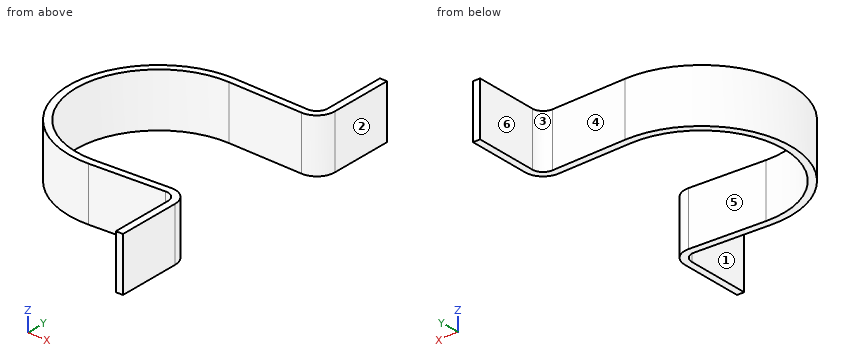
from build123d import *

# Parameters (mm, degrees)
F1_DEPTH = 15


with BuildPart() as f1:
    # F0 (on Top) → F1 (new body)
    with BuildSketch(Plane.XY):
        with BuildLine():
            ThreePointArc((0.865114, -22.983724), (-23, 0), (0.865114, 22.983724))
            Line((0.865114, 22.983724), (21.811932, 22.19528))
            ThreePointArc((21.811932, 22.19528), (25.468404, 23.59033), (27, 27.191742))
            Line((27, 27.191742), (27, 45))
            Line((27, 45), (25, 45))
            Line((25, 45), (25, 27.191742))
            ThreePointArc((25, 27.191742), (24.081043, 25.030895), (21.887159, 24.193865))
            Line((21.887159, 24.193865), (0.940341, 24.982309))
            ThreePointArc((0.940341, 24.982309), (-25, 0), (0.940341, -24.982309))
            Line((0.940341, -24.982309), (21.887159, -24.193865))
            ThreePointArc((21.887159, -24.193865), (24.081043, -25.030895), (25, -27.191742))
            Line((25, -27.191742), (25, -45))
            Line((25, -45), (27, -45))
            Line((27, -45), (27, -27.191742))
            ThreePointArc((27, -27.191742), (25.468404, -23.59033), (21.811932, -22.19528))
            Line((21.811932, -22.19528), (0.865114, -22.983724))
        make_face()
    extrude(amount=F1_DEPTH)


solid = f1.part
Can you work these out from the model? Positions are in its coordinate system, mm. Face numbers are marked on the shaded views. A direction names the side the tool comes from. Coordinates: 2 decimals unless noted, no trailing zeros. Order: outer loops, then holes, each group sorted by start corner. A loop starts at its lowest first (then second) coordinate and runs counter-clockwise, first axis right, second up. Notation, with made-up numbers: (-19, -2) -> (23, -2) arc R16 ccw to (23, 10) -> close; hole circle Ø1 at (-26, -7.5). An arc over 180 degrees is marked (long way). Use one line per item in the form item = value.
Q1. Imagine slicing it at A-A, the plane x = 0. List the corners of the cut face in (y, z) for me.
From the geometry:
outline = (-25, 0) -> (-23, 0) -> (-23, 15) -> (-25, 15) -> close; (23, 0) -> (25, 0) -> (25, 15) -> (23, 15) -> close
Q2. We'd pull the mould along X, two halves only. Please class the marked faces 1, 2 and 3: released by +X, released by -X, zero draft, split by the parting line, or undercut.
From the geometry:
face_1 = released by -X
face_2 = released by +X
face_3 = undercut
Q3. Which directions (+Z, -Z, +X, -X, +Y, -Y) give clear straight access to the entire face, cutting with the end or side of a thin tool? Please do the marked faces 4, 5 and 6.
From the geometry:
face_4 = +Z, -Z, +Y
face_5 = +Z, -Z
face_6 = +Z, -Z, -X, +Y
Q4. Imagine slicing it at B-B, the plane z = 4. List the corners of the cut face in (x, y) for me.
From the geometry:
outline = (0.87, -22.98) arc R23 cw (long way) to (0.87, 22.98) -> (21.81, 22.2) arc R5 ccw to (27, 27.19) -> (27, 45) -> (25, 45) -> (25, 27.19) arc R3 cw to (21.89, 24.19) -> (0.94, 24.98) arc R25 ccw (long way) to (0.94, -24.98) -> (21.89, -24.19) arc R3 cw to (25, -27.19) -> (25, -45) -> (27, -45) -> (27, -27.19) arc R5 ccw to (21.81, -22.2) -> close
Q5. I need wall thicknesses on L1, parallel to X at y = 36, z = 10.75; L2, parallel to Y at x = 12, z = 4; L3, parallel to Y at x = -15.5, z = 14. Which ranges of each line are inside material? Lowest first, please.
From the geometry:
L1 = 25 to 27
L2 = -24.57 to -22.56, 22.56 to 24.57
L3 = -19.62 to -16.99, 16.99 to 19.62
Q6. Imagine slicing it at C-C, the plane y = 0. List the corners of the cut face in (x, z) for me.
From the geometry:
outline = (-25, 0) -> (-23, 0) -> (-23, 15) -> (-25, 15) -> close
Q7. Will these pins go through, and if not, where does the flat tip stop? P1, Ø6, axis at y = -16.5, z = 13, coming from the +X side; P2, Ø3, axis at y = 13.5, z = 13, coming from the +X side; P3, Ø1, axis at x = 7.5, z = 3.5, coming from the -Y side; P4, Ø10, axis at x = -17, y = 5.5, coming from the -Z side.
From the geometry:
P1 = -12.2
P2 = -17.44
P3 = -24.75
P4 = through
Q8. Imagine slicing it at D-D, the plane y = -19. List the corners of the cut face in (x, z) for me, then the cut area to 3 significant figures.
From the geometry:
outline = (-16.25, 0) -> (-12.96, 0) -> (-12.96, 15) -> (-16.25, 15) -> close
area = 49.3 mm²
